```python
from build123d import *

# Parameters (mm, degrees)
SKETCH1_W           = 13.843
SKETCH1_H           = 48.133
BOSS_EXTRUDE1_DEPTH = 4.7625
SKETCH2_W           = 13.843
SKETCH2_H           = 13.843
BOSS_EXTRUDE2_DEPTH = 9.55675
SKETCH3_R           = 3.3782
CUT_EXTRUDE1_DEPTH  = 9.55675
SKETCH4_R           = 2.5527
CUT_EXTRUDE2_DEPTH  = 16.92275
SKETCH5_W           = 13.843
SKETCH5_H           = 13.843
BOSS_EXTRUDE3_DEPTH = 19.812
CUT_EXTRUDE3_DEPTH  = 19.812
SKETCH7_W           = 13.843
SKETCH7_H           = 4.7625
BOSS_EXTRUDE4_DEPTH = 70.2818
SKETCH8_W           = 13.843
SKETCH8_H           = 13.843
BOSS_EXTRUDE5_DEPTH = 29.36875
CUT_EXTRUDE4_DEPTH  = 7.62
SKETCH10_R          = 2.2
CUT_EXTRUDE5_DEPTH  = 27.51125


with BuildPart() as part:
    # Sketch1 → Boss-Extrude1 (new body)
    with BuildSketch(Plane.XY):
        with Locations((6.9215, 24.0665)):
            Rectangle(SKETCH1_W, SKETCH1_H)
    extrude(amount=BOSS_EXTRUDE1_DEPTH)

    # Sketch2 → Boss-Extrude2 (add)
    with BuildSketch(Plane.XY.offset(4.7625)):
        with Locations((6.9215, 41.2115)):
            Rectangle(SKETCH2_W, SKETCH2_H)
    extrude(amount=BOSS_EXTRUDE2_DEPTH)

    # Sketch3 → Cut-Extrude1 (cut)
    with BuildSketch(Plane(origin=(0, 0, 0), x_dir=(-1, 0, 0), z_dir=(0, 0, -1))):
        with Locations((-6.9215, 6.9215)):
            Circle(SKETCH3_R)
    extrude(amount=-CUT_EXTRUDE1_DEPTH, mode=Mode.SUBTRACT)

    # Sketch4 → Cut-Extrude2 (cut)
    with BuildSketch(Plane(origin=(0, 0, 0), x_dir=(-1, 0, 0), z_dir=(0, 0, -1))):
        with Locations((-6.9215, 41.2115)):
            Circle(SKETCH4_R)
    extrude(amount=-CUT_EXTRUDE2_DEPTH, mode=Mode.SUBTRACT)

    # Sketch5 → Boss-Extrude3 (add)
    with BuildSketch(Plane(origin=(0, 0, 0), x_dir=(-1, 0, 0), z_dir=(0, 0, -1))):
        with Locations((-6.9215, 41.2115)):
            Rectangle(SKETCH5_W, SKETCH5_H)
    extrude(amount=BOSS_EXTRUDE3_DEPTH)

    # Sketch6 → Cut-Extrude3 (cut)
    with BuildSketch(Plane(origin=(0, 0, -19.812), x_dir=(-1, 0, 0), z_dir=(0, 0, -1))):
        Polygon((-9.731894722, 46.082850851), (-12.545410948, 41.213302202), (-9.735016227, 36.341951351), (-4.111105278, 36.340149149), (-1.297589052, 41.209697798), (-4.107983773, 46.081048649), align=None)
    extrude(amount=-CUT_EXTRUDE3_DEPTH, mode=Mode.SUBTRACT)

    # Sketch7 → Boss-Extrude4 (add)
    with BuildSketch(Plane(origin=(0, 48.133, 0), x_dir=(1, 0, 0), z_dir=(0, 1, 0))):
        with Locations((6.9215, 17.43075)):
            Rectangle(SKETCH7_W, SKETCH7_H)
    extrude(amount=BOSS_EXTRUDE4_DEPTH)

    # Sketch8 → Boss-Extrude5 (add)
    with BuildSketch(Plane.XY.offset(-15.0495)):
        with Locations((6.9215, 111.4933)):
            Rectangle(SKETCH8_W, SKETCH8_H)
    extrude(amount=BOSS_EXTRUDE5_DEPTH)

    # Sketch9 → Cut-Extrude4 (cut)
    with BuildSketch(Plane(origin=(0, 0, -19.812), x_dir=(-1, 0, 0), z_dir=(0, 0, -1))):
        Polygon((-8.996554602, 115.0874), (-11.071609205, 111.4933), (-8.996554602, 107.8992), (-4.846445398, 107.8992), (-2.771390795, 111.4933), (-4.846445398, 115.0874), align=None)
    extrude(amount=-CUT_EXTRUDE4_DEPTH, mode=Mode.SUBTRACT)

    # Sketch10 → Cut-Extrude5 (cut, through all)
    with BuildSketch(Plane(origin=(0, 0, -12.192), x_dir=(-1, 0, 0), z_dir=(0, 0, -1))):
        with Locations((-6.9215, 111.4933)):
            Circle(SKETCH10_R)
    extrude(amount=-CUT_EXTRUDE5_DEPTH, mode=Mode.SUBTRACT)


solid = part.part
```
The listing builds one solid part. Answer for the finished solid, in the listing's coordinates (mm). A direction names the side the tool comes from. Round coordinates to 2 decimals unless told otherwise and drop trailing zeros. Write each loop counter-clockwise with the first axis right and the second up, starting at its lowest first coordinate (ties: lowest second). Pieces come first, ordered by that corner, then holes. Notation, with made-up numbers: (-38.75, 6.5) -> (-17.75, 6.5) arc R27 cw to (-17.75, 24.5) -> close; hole circle Ø8 at (30, 55.5). An arc over 180 degrees is marked (long way). Write item = value, one per line.
1) Section D-D on z = -13.5 is taken. Write down the section's boundary in (x, y).
Check values:
outline = (0, 34.29) -> (13.84, 34.29) -> (13.84, 48.13) -> (0, 48.13) -> close; (0, 104.57) -> (13.84, 104.57) -> (13.84, 118.41) -> (0, 118.41) -> close; hole (1.3, 41.21) -> (4.11, 36.34) -> (9.74, 36.34) -> (12.55, 41.21) -> (9.73, 46.08) -> (4.11, 46.08) -> close; hole (2.77, 111.49) -> (4.85, 107.9) -> (9, 107.9) -> (11.07, 111.49) -> (9, 115.09) -> (4.85, 115.09) -> close
2) Section A-A on z = -3.5 is taken. Write down the section's boundary in (x, y).
Check values:
outline = (0, 34.29) -> (13.84, 34.29) -> (13.84, 48.13) -> (0, 48.13) -> close; (0, 104.57) -> (13.84, 104.57) -> (13.84, 118.41) -> (0, 118.41) -> close; hole (1.3, 41.21) -> (4.11, 36.34) -> (9.74, 36.34) -> (12.55, 41.21) -> (9.73, 46.08) -> (4.11, 46.08) -> close; hole circle Ø4.4 at (6.92, 111.49)
3) Section C-C on x = 6.75 is taken. Give the number of separate pieces and of enclosed holes in the cut face, plus the area to 3 significant figures.
Check values:
separate_pieces = 4
enclosed_holes = 0
area = 908 mm²
4) Section B-B on z = 2 is taken. Write down the section's boundary in (x, y).
Check values:
outline = (0, 0) -> (13.84, 0) -> (13.84, 48.13) -> (0, 48.13) -> close; (0, 104.57) -> (13.84, 104.57) -> (13.84, 118.41) -> (0, 118.41) -> close; hole circle Ø6.76 at (6.92, 6.92); hole circle Ø5.11 at (6.92, 41.21); hole circle Ø4.4 at (6.92, 111.49)
5) Given pin 1 (5 mm diameter, centred on x = 7.5, z = 9, fed in from -Y); pin 2 (1.5 mm diameter, centred on y = 45.5, z = 9, fed in from -X); pin 3 (1 mm diameter, centred on y = 14.5, z = 7, fed in from +X); pin 4 (1.5 mm diameter, centred on x = 7.5, y = 22.5, fed in from -Z), each flat-ended and moving along its own axis, determine where each tip first touches the part or whether it passes through.
Check values:
pin_1 = 34.29
pin_2 = 0
pin_3 = through
pin_4 = 0
6) Which of the six approach directions +Z, -Z, +X, -X, +Y, -Y give full straight-line access (tool end or side, diameter ignored) to faces 4 (the flat face through (2.683, 43.611, -10.045)), 5 (the flat face through (7, 104.572, -1)), 6 (the flat face through (7, 44, 14.319))?
Check values:
face_4 = -Z
face_5 = +Z, +X, -X
face_6 = +Z, +X, -X, +Y, -Y
7) Straight lines are drawn through the part: line 1 along Y through (x, z) = (7, -6.5); line 2 along Y through (x, z) = (3.75, 13); line 3 along Y through (x, z) = (12, 1). For each, find the intervals that lie inside material, in ascending order. Write a range as [from, to].
Check values:
line_1 = [34.29, 36.34], [46.08, 48.13], [104.57, 109.29], [113.69, 118.41]
line_2 = [34.29, 48.13], [104.57, 118.41]
line_3 = [0, 48.13], [104.57, 118.41]
8) For a pull along Y with two mould halves and no side action, classify faces 1 (the cylindrical face through (7.208, 113.675, 0.878)), 2 (the flat face through (7, 17, 0)), 3 (the flat face through (7, 34.29, -10)) as released by +Y, released by -Y, zero draft, split by the parting line, or undercut.
Check values:
face_1 = undercut
face_2 = zero draft
face_3 = released by -Y
